Verification items for the finished model (mm, model axes). Face numbers are marked on the shaded views. A direction names the side the tool comes from. Give positions to 0.01 mm unless a question says otherwise; leave off trailing zeros. Order: outer loops, then holes, each group sorted by start corner. A loop starts at its lowest first (then second) coordinate and runs counter-clockwise, first axis right, second up. Notation, with made-up numbers: (78.25, 46) -> (108.25, 46) arc R21 ccw to (108.25, 51) -> close; hole circle Ø6 at (10, 49). An arc over 180 degrees is marked (long way). Return JSON: item names as keys, results as strings. Group by question number.
(1) Cross-section at B-B on y = 25. Enter the section's corners in (x, z), then the cut area to 3 significant figures.
(2) Cross-section at A-A on x = 0. Enter the section's corners in (y, z), then the cut area to 3 significant figures.
(3) Cross-section at D-D on z = -6.5. Enter the section's corners in (x, y).
(4) Thickness scan on line 1 along Y through (x, z) = (0, -29.9); line 2 along X through (y, z) = (33, -29); line 3 along X through (y, z) = (6, -16). Record the ranges inside material, lowest first.
(5) Depth check by flat-ended pin: pin 1 Ø0.6 at (x, z) = (-9.5, -16) entering from +Y; pin 2 Ø5 at (x, z) = (1, -9) entering from +Y; pin 3 Ø1 at (x, y) = (-2.5, 4.5) entering from +Z; pin 4 Ø6 at (y, z) = (23.5, -12.5) entering from -X. Enter the tip coordinate at first touch or a pass-through.
(6) Tool access check on the marked faces 4, 5 and 6. Record the directions out of +Z, -Z, +X, -X, +Y, -Y that give a thin tool (end or side, any length) a straight path to the whole face; none if there is none.
(7) Cross-section at C-C on x = -8. Enter the section's corners in (y, z), then the cut area to 3 significant figures.
(8) Release check for a two-part mould opening along X. For the marked faces 1, 2 and 3 record: pulls with the +X half, pulls with the -X half, needs draft (parallel to the pull), parting line crosses it, or undercut.
from build123d import *

# Parameters (mm, degrees)
BOSS_EXTRUDE1_DEPTH = 10
SHELL1_T            = -1.25
RIB1_REACH          = 57.985
SKETCH4_WALL_W      = 164.251441786
SKETCH4_WALL_H      = 1.25
SKETCH5_W           = 7.5
SKETCH5_H           = 22.5
BOSS_EXTRUDE2_DEPTH = 2.5
SKETCH6_R           = 1.25
CUT_EXTRUDE1_DEPTH  = 52.599418601


with BuildPart() as part:
    # Sketch1 → Boss-Extrude1 (new, symmetric)
    with BuildSketch(Plane(origin=(0, 0, 0), x_dir=(0, 0, -1), z_dir=(1, 0, 0))):
        Polygon((0, 0), (31.25, 0), (31.25, 42.5), (26.25, 42.5), (26.25, 5), (0, 5), align=None)
    extrude(amount=BOSS_EXTRUDE1_DEPTH, both=True)

    # Shell1
    shell1_openings = [part.faces().sort_by_distance(p)[0] for p in [
        (0, 5, -13.125),
        (0, 23.75, -26.25),
        (0, 42.5, -28.75),
        (0, 2.5, 0),
    ]]
    offset(amount=SHELL1_T, openings=shell1_openings, kind=Kind.INTERSECTION)

    # Sketch4 wall → Rib1 (add, up to next)
    with BuildSketch(Plane(origin=(-8.75, 20.625, -16.875), x_dir=(0, 0.82039816677, -0.571792661688), z_dir=(0, 0.571792661688, 0.82039816677)), mode=Mode.PRIVATE) as rib1_sk1:
        with Locations((0, -0.625)):
            Rectangle(SKETCH4_WALL_W, SKETCH4_WALL_H)
    rib1_tool1 = extrude(rib1_sk1.sketch, amount=-RIB1_REACH, mode=Mode.PRIVATE) - part.part
    rib1 = rib1_tool1.solids().sort_by_distance((-8.75, 20.625, -16.875))[0]
    add(rib1)

    # Mirror1: Rib1 across plane
    add(rib1.mirror(Plane(origin=(0, 0, 0), x_dir=(0, 0, 1), z_dir=(1, 0, 0))))

    # Sketch5 → Boss-Extrude2 (add)
    with BuildSketch(Plane.XY.offset(-30)):
        with Locations((0, 28.206521739)):
            Rectangle(SKETCH5_W, SKETCH5_H)
    extrude(amount=BOSS_EXTRUDE2_DEPTH)

    # Sketch6 → Cut-Extrude1 (cut, through all)
    with BuildSketch(Plane.XY.offset(-27.5)):
        with Locations((0, 35)):
            Circle(SKETCH6_R)
        with Locations((0, 25)):
            Circle(SKETCH6_R)
    extrude(amount=-CUT_EXTRUDE1_DEPTH, mode=Mode.SUBTRACT)


solid = part.part
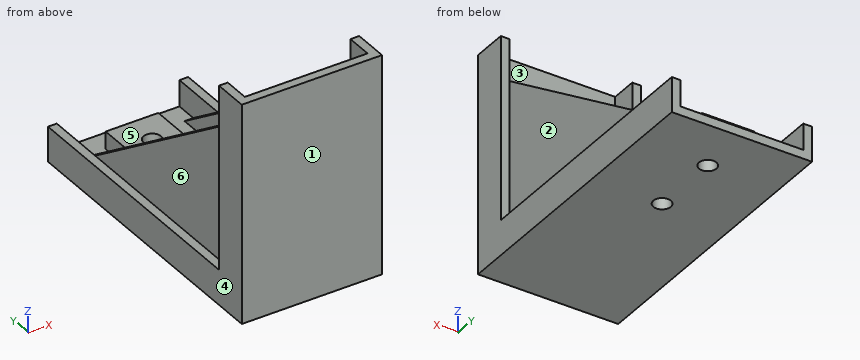
Verdict:
{
 "1": {"outline": "(-10, -31.25) -> (-1.25, -31.25) -> (-1.25, -27.5) -> (-3.75, -27.5) -> (-3.75, -30) -> (-7.5, -30) -> (-7.5, -19.92) -> (-8.75, -19.92) -> (-8.75, -26.25) -> (-10, -26.25) -> close; (1.25, -31.25) -> (10, -31.25) -> (10, -26.25) -> (8.75, -26.25) -> (8.75, -19.92) -> (7.5, -19.92) -> (7.5, -30) -> (3.75, -30) -> (3.75, -27.5) -> (1.25, -27.5) -> close", "area": "68.9 mm²"},
 "2": {"outline": "(0, -31.25) -> (23.75, -31.25) -> (23.75, -27.5) -> (16.96, -27.5) -> (16.96, -30) -> (1.25, -30) -> (1.25, 0) -> (0, 0) -> close; (26.25, -31.25) -> (33.75, -31.25) -> (33.75, -27.5) -> (26.25, -27.5) -> close; (36.25, -31.25) -> (42.5, -31.25) -> (42.5, -30) -> (39.46, -30) -> (39.46, -27.5) -> (36.25, -27.5) -> close", "area": "128 mm²"},
 "3": {"outline": "(-10, 0) -> (10, 0) -> (10, 5) -> (8.75, 5) -> (8.75, 5.74) -> (7.5, 5.74) -> (7.5, 1.25) -> (-7.5, 1.25) -> (-7.5, 5.74) -> (-8.75, 5.74) -> (-8.75, 5) -> (-10, 5) -> close"},
 "4": {"line 1": "0 to 1.25, 16.96 to 23.75, 26.25 to 33.75, 36.25 to 39.46", "line 2": "-10 to -7.5, -3.75 to 3.75, 7.5 to 10", "line 3": "-8.75 to -7.5, 7.5 to 8.75"},
 "5": {"pin 1": "y = 5", "pin 2": "y = 1.25", "pin 3": "z = -30", "pin 4": "through"},
 "6": {"face 4": "+Z, -Z, -X, +Y, -Y", "face 5": "+Z, +Y", "face 6": "+Z, -X, +Y"},
 "7": {"outline": "(0, -31.25) -> (42.5, -31.25) -> (42.5, -30) -> (39.46, -30) -> (1.25, -3.37) -> (1.25, 0) -> (0, 0) -> close", "area": "599 mm²"},
 "8": {"face 1": "needs draft", "face 2": "pulls with the +X half", "face 3": "undercut"}
}
